Input: part model. Units: mm. Frame: model coordinates. Coordinates: 2 decimals unless noted, no trailing zeros. Loops run counter-clockwise (first coordinate to the right, second up) from the corner with the lowest first, then second, coordinate; pieces in that order, holes last. Notation, with made-up numbers: M 50.25,-23 L 62.25,-23 A21 ccw 62.25,-7 Z; hole C 81,-8 d1. An arc over 180 degrees is marked long. Use a Markdown table: item, result. Add a question column.
1. Section A-A on x = 0. Output: boundary loops of the cut face in (y, z).
2. Section B-B on z = -64.5. Output: boundary loops of the cut face in (x, y), then the cut area to 3 significant figures.
3. Pin query (flat end, axial travel): pin 1 (4 mm diameter, centred on x = 0, y = -3, fed in from +Z); pin 2 (3 mm diameter, centred on x = 1, z = -1.5, fed in from -Y). Return the tip coordinate at first contact, or that it passes through.
4. Line query: L1, parallel to Y at x = 0, z = -113.9; L2, parallel to Z at x = 3, y = 1.5; L3, parallel to X at y = -3, z = 113.25. Output: solid intervals per line, ascending. Write a range as [from, to].
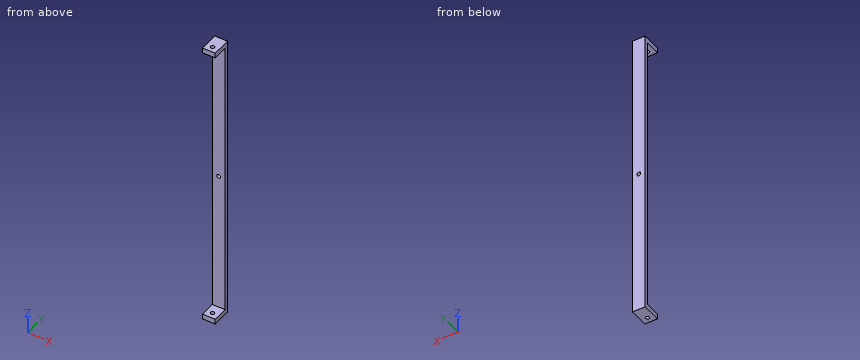
```python
from build123d import *

# Parameters (mm, degrees)
CROQUIS1_W              = 10
CROQUIS1_H              = 15
CROQUIS1_R              = 1.5
SALIENTE_EXTRUIR1_DEPTH = 115
CROQUIS2_W              = 222
CROQUIS2_H              = 12
CORTAR_EXTRUIR1_DEPTH   = 11
CROQUIS3_R              = 1.5
CORTAR_EXTRUIR2_DEPTH   = 10


with BuildPart() as part:
    # Croquis1 → Saliente-Extruir1 (new body, symmetric)
    with BuildSketch(Plane.XY):
        Rectangle(CROQUIS1_W, CROQUIS1_H)
        with Locations((0, -3)):
            Circle(CROQUIS1_R, mode=Mode.SUBTRACT)
    extrude(amount=SALIENTE_EXTRUIR1_DEPTH, both=True)

    # Croquis2 → Cortar-Extruir1 (cut, through all)
    with BuildSketch(Plane.ZY.offset(5)):
        with Locations((0, -1.5)):
            Rectangle(CROQUIS2_W, CROQUIS2_H)
    extrude(amount=-CORTAR_EXTRUIR1_DEPTH, mode=Mode.SUBTRACT)

    # Croquis3 → Cortar-Extruir2 (cut)
    with BuildSketch(Plane(origin=(0, 7.5, 0), x_dir=(1, 0, 0), z_dir=(0, 1, 0))):
        Circle(CROQUIS3_R)
    extrude(amount=-CORTAR_EXTRUIR2_DEPTH, mode=Mode.SUBTRACT)


solid = part.part
```
Answers below:
| question | item | result |
|---|---|---|
| 1 | outline | M -7.5,-115 L -4.5,-115 L -4.5,-111 L -7.5,-111 Z; M -7.5,111 L -4.5,111 L -4.5,115 L -7.5,115 Z; M -1.5,-115 L 7.5,-115 L 7.5,-1.5 L 4.5,-1.5 L 4.5,-111 L -1.5,-111 Z; M -1.5,111 L 4.5,111 L 4.5,1.5 L 7.5,1.5 L 7.5,115 L -1.5,115 Z |
| 2 | outline | M -5,4.5 L 5,4.5 L 5,7.5 L -5,7.5 Z |
| 2 | area | 30.0 mm² |
| 3 | pin 1 | stops at z = 115 |
| 3 | pin 2 | stops at y = 4.5 |
| 4 | L1 | y = [-7.5, -4.5], [-1.5, 7.5] |
| 4 | L2 | z = [-115, -111], [111, 115] |
| 4 | L3 | x = [-5, -1.5], [1.5, 5] |
